Study the drawing (mm; zero at the part's minimum x, y, z) and answer. Coordinates: 2 decimals unless noted, no trailing zeros. Loops run counter-clockwise (first coordinate to the right, second up) from the corner with the lowest first, then second, coordinate; pieces in that order, holes last. Notation, with made-up numbers: (11, 19.25) - (38, 19.25) arc R18 ccw to (38, 33.25) - close; hole circle Ø10 at (68.25, 64). An arc over 180 degrees is marked (long way). Use CSV: the item, a comma, the result in double quotes.
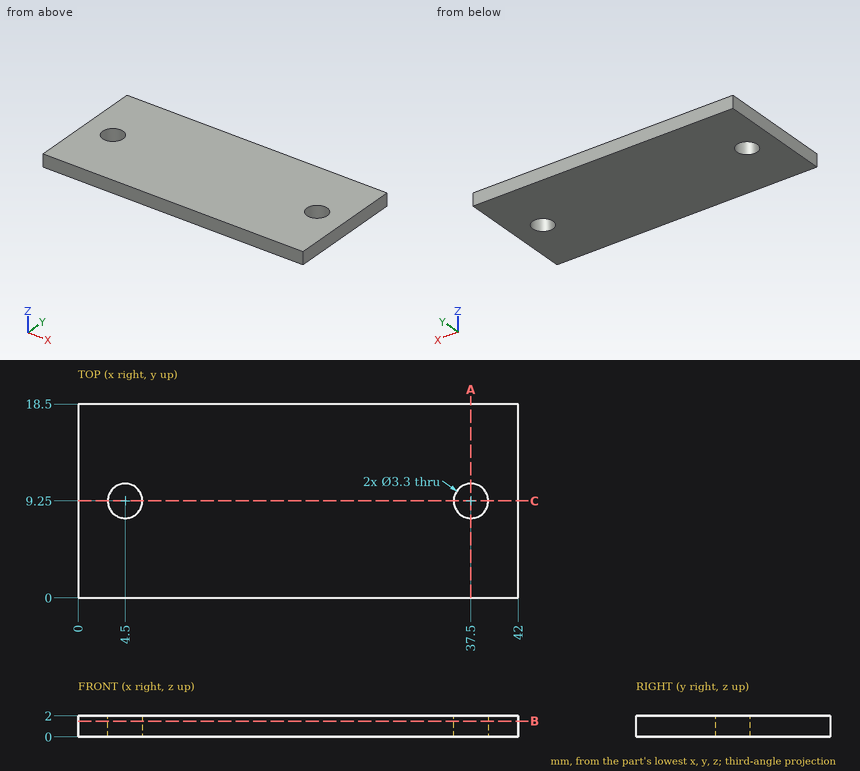
Q1. The part is cut by section A-A on x = 37.5. Determine the outline of the cut face in (y, z), and give its area (3 significant figures).
Reported:
outline,"(0, 0) - (7.6, 0) - (7.6, 2) - (0, 2) - close; (10.9, 0) - (18.5, 0) - (18.5, 2) - (10.9, 2) - close"
area,"30.4 mm²"
Q2. The part is cut by section B-B on z = 1.5. Determine the outline of the cut face in (x, y), and give its area (3 significant figures).
Reported:
outline,"(0, 0) - (42, 0) - (42, 18.5) - (0, 18.5) - close; hole circle Ø3.3 at (4.5, 9.25); hole circle Ø3.3 at (37.5, 9.25)"
area,"760 mm²"
Q3. The part is cut by section C-C on y = 9.25. Determine the outline of the cut face in (x, z), and give its area (3 significant figures).
Reported:
outline,"(0, 0) - (2.85, 0) - (2.85, 2) - (0, 2) - close; (6.15, 0) - (35.85, 0) - (35.85, 2) - (6.15, 2) - close; (39.15, 0) - (42, 0) - (42, 2) - (39.15, 2) - close"
area,"70.8 mm²"
Q4. Find the intervals of material crossed by probe 1 along Y at (x, z) = (4.5, 1.1); probe 2 along X at (y, z) = (10, 1.15); probe 3 along Y at (x, z) = (4, 1.5), in increasing order. Write a range as [from, to].
Reported:
probe 1,"y = [0, 7.6], [10.9, 18.5]"
probe 2,"x = [0, 3.03], [5.97, 36.03], [38.97, 42]"
probe 3,"y = [0, 7.68], [10.82, 18.5]"
Q5. Given P1, Ø2, axis at x = 4.5, y = 9.25, coming from the +Z side, flat-ended and moving along its own axis, determine where the tip first touches the part or whether it passes through.
Reported:
P1,"passes through"
